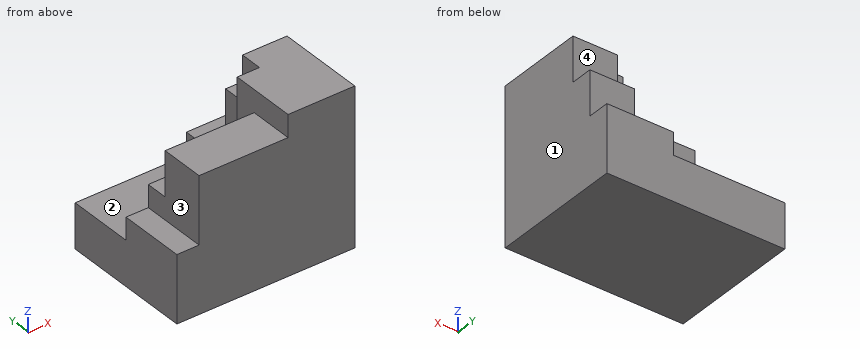
```python
from build123d import *

# Parameters (mm, degrees)
SKETCH1_W           = 8
SKETCH1_H           = 7
BOSS_EXTRUDE1_DEPTH = 6
CUT_EXTRUDE1_DEPTH  = 60
CUT_EXTRUDE2_DEPTH  = 3
SKETCH5_W           = 4
SKETCH5_H           = 2
CUT_EXTRUDE3_DEPTH  = 1
SKETCH6_W           = 3.001059972
SKETCH6_H           = 4.860975679
CUT_EXTRUDE4_DEPTH  = 1
SKETCH7_W           = 2
SKETCH7_H           = 2
CUT_EXTRUDE5_DEPTH  = 1


with BuildPart() as part:
    # Sketch1 → Boss-Extrude1 (new body)
    with BuildSketch(Plane(origin=(0, 0, 0), x_dir=(1, 0, 0), z_dir=(0, 1, 0))):
        Rectangle(SKETCH1_W, SKETCH1_H)
    extrude(amount=BOSS_EXTRUDE1_DEPTH)

    # Sketch2 → Cut-Extrude1 (cut)
    with BuildSketch(Plane(origin=(0, 6, 0), x_dir=(1, 0, 0), z_dir=(0, 1, 0))):
        Polygon((-4, 0.5), (-3, 0.5), (-3, -2.5), (1, -2.5), (1, -3.5), (-4, -3.5), align=None)
    extrude(amount=-CUT_EXTRUDE1_DEPTH, mode=Mode.SUBTRACT)

    # Sketch4 → Cut-Extrude2 (cut)
    with BuildSketch(Plane(origin=(0, 6, 0), x_dir=(1, 0, 0), z_dir=(0, 1, 0))):
        Polygon((-4, 1.5), (1, 1.5), (1, 0.5), (2, 0.5), (2, -4.455907127), (-4, -3.689508324), align=None)
    extrude(amount=-CUT_EXTRUDE2_DEPTH, mode=Mode.SUBTRACT)

    # Sketch5 → Cut-Extrude3 (cut)
    with BuildSketch(Plane(origin=(0, 3, 0), x_dir=(1, 0, 0), z_dir=(0, 1, 0))):
        with Locations((-1, -1.5)):
            Rectangle(SKETCH5_W, SKETCH5_H)
    extrude(amount=-CUT_EXTRUDE3_DEPTH, mode=Mode.SUBTRACT)

    # Sketch6 → Cut-Extrude4 (cut)
    with BuildSketch(Plane(origin=(0, 6, 0), x_dir=(1, 0, 0), z_dir=(0, 1, 0))):
        with Locations((3.500529986, -1.93048784)):
            Rectangle(SKETCH6_W, SKETCH6_H)
    extrude(amount=-CUT_EXTRUDE4_DEPTH, mode=Mode.SUBTRACT)

    # Sketch7 → Cut-Extrude5 (cut)
    with BuildSketch(Plane(origin=(0, 5, 0), x_dir=(1, 0, 0), z_dir=(0, 1, 0))):
        with Locations((3, -2.5)):
            Rectangle(SKETCH7_W, SKETCH7_H)
    extrude(amount=-CUT_EXTRUDE5_DEPTH, mode=Mode.SUBTRACT)


solid = part.part
```
Work out the finished part from the listing and answer in its coordinate system (mm). Face numbers are marked on the shaded views. A direction names the side the tool comes from. Coordinates: 2 decimals unless noted, no trailing zeros. Loops run counter-clockwise (first coordinate to the right, second up) from the corner with the lowest first, then second, coordinate; pieces in that order, holes last. Notation, with made-up numbers: M -9,-19 L 22,-19 A34 ccw 22,15 Z; hole C 41.5,1 d9. An arc over 180 degrees is marked long. Use CSV: the item, a comma, the result in double quotes. Start each with the question number.
(1) Find section D-D, the plane z = 3. Give the vertices of the cut face in (x, y).
(2) Find section C-C, the plane y = 5.45. Give the vertices of the cut face in (x, z).
(3) Given pin 1 Ø1.5 at (y, z) = (1, 1) entering from -X; pin 2 Ø0.5 at (x, y) = (-3.5, 1.5) entering from +Z; pin 3 Ø1.5 at (x, y) = (2, 5) entering from +Z, each flat-ended and moving along its own axis, determine where each tip first touches the part or whether it passes through.
(4) Find section B-B, the plane z = 1. Give the vertices of the cut face in (x, y), then the cut area to 3 significant figures.
(5) Consider line 1 (Y direction, x = -2, z = 1.5); line 2 (Y direction, x = -2.75, z = -1.25); line 3 (Z direction, x = -2.75, y = 3.3). Determine where each line is inside the solid, lowest interval first.
(6) For the marked faces 1, 2, 3 and 4, determine the directions among +Z, -Z, +X, -X, +Y, -Y from which every point of the face is accessible in a straight line to the end or side of a thin tool.
(7) Find section A-A, the plane x = 0.5. Give the vertices of the cut face in (y, z).
Recorded:
1,outline,"M 1,0 L 4,0 L 4,4 L 2,4 L 2,3 L 1,3 Z"
2,outline,"M -4,-3.5 L 4,-3.5 L 4,-0.5 L 1,-0.5 L 1,-1.5 L -4,-1.5 Z"
3,pin 1,"stops at x = -3"
3,pin 2,"stops at z = -0.5"
3,pin 3,"stops at z = 1.5"
4,outline,"M -3,0 L 4,0 L 4,5 L 2,5 L 2,3 L 1,3 L 1,2 L -3,2 Z"
4,area,"21.0 mm^2"
5,line 1,"y = 0 to 2"
5,line 2,"y = 0 to 3"
5,line 3,"z = -3.5 to -1.5"
6,face 1,"+Z, -Z, +X, +Y, -Y"
6,face 2,"+Z, -X, +Y"
6,face 3,"+Z, -X, +Y, -Y"
6,face 4,"+Z, +X, -X, +Y"
7,outline,"M 0,-3.5 L 6,-3.5 L 6,-1.5 L 3,-1.5 L 3,0.5 L 2,0.5 L 2,2.5 L 0,2.5 Z"
